```python
from build123d import *

# Parameters (mm, degrees)
SKETCH1_R                       = 2.5
BOSS_EXTRUDE1_DEPTH             = 15
SKETCH2_R                       = 1
CUT_EXTRUDE1_DEPTH              = 16.411035007
TAP_DRILL_FOR_M4X0_7_TAP1_D     = 3.3
TAP_DRILL_FOR_M4X0_7_TAP1_DEPTH = 11
TAP_DRILL_FOR_M4X0_7_TAP1_TIP   = 0.991420021
CHAMFER1_SIZE                   = 0.4
CHAMFER1_SIZE2                  = 0.230940108
CHAMFER2_SIZE                   = 0.5
CHAMFER2_SIZE2                  = 0.866025404


with BuildPart() as part:
    # Sketch1 → Boss-Extrude1 (new body)
    with BuildSketch(Plane.XY):
        Circle(SKETCH1_R)
    extrude(amount=BOSS_EXTRUDE1_DEPTH)

    # Sketch2 → Cut-Extrude1 (cut, through all)
    with BuildSketch(Plane(origin=(0, 0, 0), x_dir=(-1, 0, 0), z_dir=(0, 0, -1))):
        Circle(SKETCH2_R)
    extrude(amount=-CUT_EXTRUDE1_DEPTH, mode=Mode.SUBTRACT)

    # Tap Drill for M4x0.7 Tap1
    with Locations(Plane(origin=(0, 0, 0), x_dir=(-1, 0, 0), z_dir=(0, 0, -1))):
        with Locations((0, 0)):
            Hole(TAP_DRILL_FOR_M4X0_7_TAP1_D / 2, depth=TAP_DRILL_FOR_M4X0_7_TAP1_DEPTH)
            with Locations((0, 0, -(TAP_DRILL_FOR_M4X0_7_TAP1_DEPTH + TAP_DRILL_FOR_M4X0_7_TAP1_TIP / 2))):  # 118° drill point
                Cone(0, TAP_DRILL_FOR_M4X0_7_TAP1_D / 2, TAP_DRILL_FOR_M4X0_7_TAP1_TIP, mode=Mode.SUBTRACT)

    # Chamfer1
    chamfer1_edges = [part.edges().sort_by_distance(p)[0] for p in [
        (-2.5, 0, 15),
    ]]
    chamfer1_side = [part.faces().sort_by_distance(p)[0] for p in [
        (-2.5, 0, 7.5),
    ]]
    chamfer(chamfer1_edges, length=CHAMFER1_SIZE, length2=CHAMFER1_SIZE2, reference=chamfer1_side[0])

    # Chamfer2
    chamfer2_edges = [part.edges().sort_by_distance(p)[0] for p in [
        (-1.65, 0, 0),
    ]]
    chamfer2_side = [part.faces().sort_by_distance(p)[0] for p in [
        (-2.429289322, 0, 0),
    ]]
    chamfer(chamfer2_edges, length=CHAMFER2_SIZE, length2=CHAMFER2_SIZE2, reference=chamfer2_side[0])


solid = part.part
```
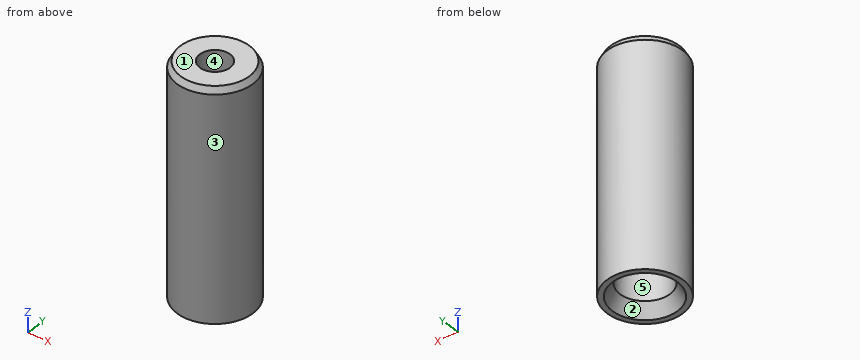
Input: part model. Units: mm. Frame: model coordinates. Face numbers are marked on the shaded views. A direction names the side the tool comes from. Give positions to 0.01 mm unless a question says otherwise; leave off trailing zeros. Order: outer loops, then holes, each group sorted by start corner. A loop starts at its lowest first (then second) coordinate and runs counter-clockwise, first axis right, second up. Notation, with made-up numbers: (-38, 61.25) - (-8, 61.25) arc R13 ccw to (-8, 76.25) - close; hole circle Ø1 at (13.25, 34). An arc over 180 degrees is marked (long way). One line per item, written item: value.
1. Cut plane A-A, the plane y = 0. Output: boundary loops of the cut face in (x, z), and give its area (3 significant figures).
Determined:
outline: (-2.5, 0) - (-2.15, 0) - (-1.65, 0.87) - (-1.65, 11) - (-1, 11.39) - (-1, 15) - (-2.27, 15) - (-2.5, 14.6) - close; (1, 11.39) - (1.65, 11) - (1.65, 0.87) - (2.15, 0) - (2.5, 0) - (2.5, 14.6) - (2.27, 15) - (1, 15) - close
area: 29.9 mm2
2. Reachability of the marked faces 4 and 5 from +Z, -Z, +X, -X, +Y, -Y: full face, straight path, thin tool, end or side. Return the list, or none.
Determined:
face 4: +Z, -Z
face 5: -Z
3. Draft query along Y for the marked faces 1, 2 and 3. Return one class per face: released by +Y, released by -Y, zero draft, split by the parting line, or undercut.
Determined:
face 1: zero draft
face 2: undercut
face 3: split by the parting line
4. Cut plane C-C, the plane z = 4. Output: boundary loops of the cut face in (x, y), and give its area (3 significant figures).
Determined:
outline: circle Ø5 at (0, 0); hole circle Ø3.3 at (0, 0)
area: 11.1 mm2
5. Pin query (flat end, axial travel): pin 1 Ø2.5 at (x, y) = (0, 0) entering from -Z. Return the tip coordinate at first contact, or that it passes through.
Determined:
pin 1: z = 11.24
6. Line query: probe 1 along Y at (x, z) = (0, 1.5); probe 2 along Y at (x, z) = (0, 12.55); probe 3 along X at (y, z) = (1.3, 1.5). Output: solid intervals per line, ascending.
Determined:
probe 1: -2.5 to -1.65, 1.65 to 2.5
probe 2: -2.5 to -1, 1 to 2.5
probe 3: -2.14 to -1.02, 1.02 to 2.14
7. Cut plane D-D, the plane z = 11.75. Output: boundary loops of the cut face in (x, y), and give its area (3 significant figures).
Determined:
outline: circle Ø5 at (0, 0); hole circle Ø2 at (0, 0)
area: 16.5 mm2
